Check sheet for the modelled part. Datum: model origin and axes. Units: mm. Face numbers are marked on the shaded views. A direction names the side the tool comes from. Round coordinates to 2 decimals unless told otherwise and drop trailing zeros. Loops run counter-clockwise (first coordinate to the right, second up) from the corner with the lowest first, then second, coordinate; pieces in that order, holes last. Notation, with made-up numbers: (-4.75, 44) - (7.25, 44) arc R29 cw to (7.25, 71) - close; hole circle Ø1 at (35.25, -3.5). An arc over 180 degrees is marked (long way). Put each result on its own line as item: value. Start each with the question number.
Item 1: Gauge pin test, flat ends, axial feed: pin 1 Ø2.5 at (x, y) = (41.5, -22) entering from -Z; pin 2 Ø2.5 at (x, y) = (40.4, -23.75) entering from -Z; pin 3 Ø1.5 at (y, z) = (-18, 0) entering from +X; pin 4 Ø1.5 at (x, z) = (48.5, 2.5) entering from +Y. Record the tip position at first contact, or that the pin passes through.
Item 2: Material ranges on line 1 along Y through (x, z) = (40.4, 1.3) (3 decimals); line 2 along Y through (x, z) = (40.4, -0.25); line 3 along Z through (x, y) = (41.5, -15.25), recorded low to high.
Item 3: Section check A-A, the plane y = -23.75. Record the cut outline in (x, z) (3 decimals).
Item 4: Section check B-B, the plane x = 40.4. Record the cut outline in (y, z) (3 decimals).
Item 5: Section check C-C, the plane z = 0.7. Record the cut outline in (x, y) (3 decimals), and give its area (3 significant figures).
Item 6: Draft check along Y on the marked faces 3, 4 and 5. Enter one of: pulls with the +Y half, pulls with the -Y half, needs draft (parallel to the pull), parting line crosses it, or undercut.
Item 7: Tool access check on the marked faces 1 and 2. Record the directions out of +Z, -Z, +X, -X, +Y, -Y that give a thin tool (end or side, any length) a straight path to the whole face; none if there is none.
from build123d import *

# Parameters (mm, degrees)
SKETCH2_R           = 5.5
SKETCH2_R_2         = 3.923
BOSS_EXTRUDE1_DEPTH = 0.5
SKETCH3_R           = 13
SKETCH3_R_2         = 5.5
SKETCH3_R_3         = 3.923
BOSS_EXTRUDE2_DEPTH = 3
SKETCH4_R           = 1.435
CUT_EXTRUDE1_DEPTH  = 65.893162175
CHAMFER1_SIZE       = 1.27
CHAMFER1_SIZE2      = 2.199704526


with BuildPart() as part:
    # Sketch2 → Boss-Extrude1 (new body)
    with BuildSketch(Plane.XY.offset(-0.5)):
        with Locations((40.399999972, -23.75)):
            Circle(SKETCH2_R)
        with Locations((40.399999972, -23.75)):
            Circle(SKETCH2_R_2, mode=Mode.SUBTRACT)
    extrude(amount=BOSS_EXTRUDE1_DEPTH)

    # Sketch3 → Boss-Extrude2 (add)
    with BuildSketch(Plane.XY):
        with Locations((40.399999972, -23.75)):
            Circle(SKETCH3_R)
        with Locations((40.399999972, -23.75)):
            Circle(SKETCH3_R_2, mode=Mode.SUBTRACT)
        with Locations((40.399999972, -23.75)):
            Circle(SKETCH3_R_2)
        with Locations((40.399999972, -23.75)):
            Circle(SKETCH3_R_3, mode=Mode.SUBTRACT)
        with Locations((40.399999972, -23.75)):
            Circle(SKETCH3_R_3)
    extrude(amount=BOSS_EXTRUDE2_DEPTH)

    # Sketch4 → Cut-Extrude1 (cut, through all)
    with BuildSketch(Plane(origin=(0, 0, 0), x_dir=(-1, 0, 0), z_dir=(0, 0, -1))):
        with Locations((-40.399999972, -23.75)):
            Circle(SKETCH4_R)
    extrude(amount=-CUT_EXTRUDE1_DEPTH, mode=Mode.SUBTRACT)

    # Chamfer1
    chamfer1_edges = [part.edges().sort_by_distance(p)[0] for p in [
        (27.399999972, -23.75, 3),
    ]]
    chamfer1_side = [part.faces().sort_by_distance(p)[0] for p in [
        (27.399999972, -23.75, 1.5),
    ]]
    chamfer(chamfer1_edges, length=CHAMFER1_SIZE, length2=CHAMFER1_SIZE2, reference=chamfer1_side[0])


solid = part.part
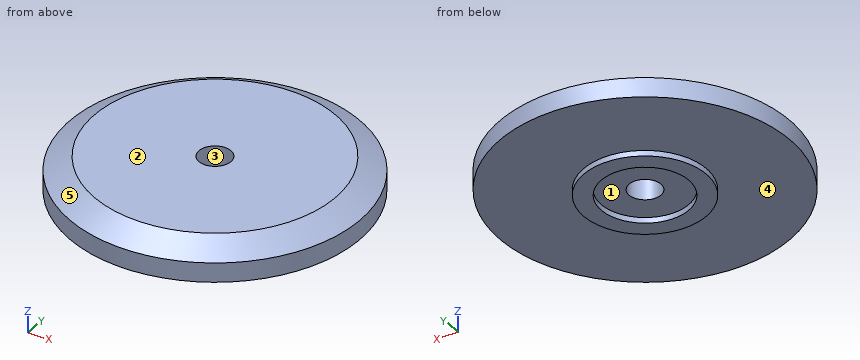
Check result:
1. pin 1: z = 0
1. pin 2: through
1. pin 3: x = 52.4
1. pin 4: y = -13.52
2. line 1: -36.75 to -25.185, -22.315 to -10.75
2. line 2: -29.25 to -27.67, -19.83 to -18.25
2. line 3: 0 to 3
3. outline: (27.4, 0) - (34.9, 0) - (34.9, -0.5) - (36.477, -0.5) - (36.477, 0) - (38.965, 0) - (38.965, 3) - (29.6, 3) - (27.4, 1.73) - close; (41.835, 0) - (44.323, 0) - (44.323, -0.5) - (45.9, -0.5) - (45.9, 0) - (53.4, 0) - (53.4, 1.73) - (51.2, 3) - (41.835, 3) - close
4. outline: (-36.75, 0) - (-29.25, 0) - (-29.25, -0.5) - (-27.673, -0.5) - (-27.673, 0) - (-25.185, 0) - (-25.185, 3) - (-34.55, 3) - (-36.75, 1.73) - close; (-22.315, 0) - (-19.827, 0) - (-19.827, -0.5) - (-18.25, -0.5) - (-18.25, 0) - (-10.75, 0) - (-10.75, 1.73) - (-12.95, 3) - (-22.315, 3) - close
5. outline: circle Ø26 at (40.4, -23.75); hole circle Ø2.87 at (40.4, -23.75)
5. area: 524 mm²
6. face 3: undercut
6. face 4: needs draft
6. face 5: parting line crosses it
7. face 1: -Z
7. face 2: +Z, +X, -X, +Y, -Y
